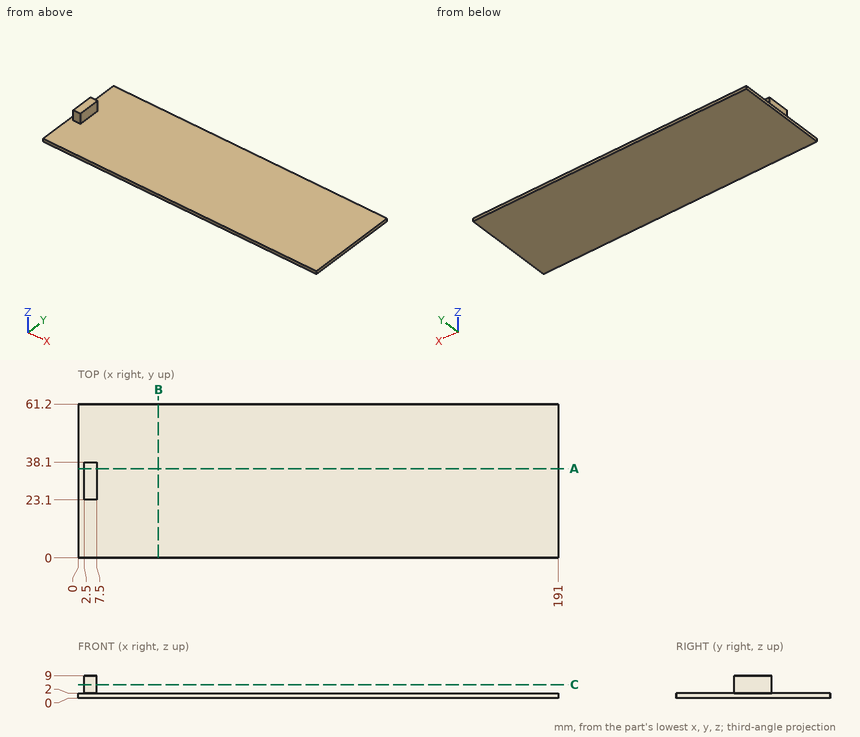
Check sheet for the drawn part. Datum: minimum x, y, z corner. Units: mm. Give positions to 0.01 mm unless a question says otherwise; leave off trailing zeros. Order: outer loops, then holes, each group sorted by start corner. A loop starts at its lowest first (then second) coordinate and runs counter-clockwise, first axis right, second up.
1. Sectioned sample at A-A (y = 35.5). Record the boundary of the cut face in (x, z).
Completed:
outline: (0, 0) - (191, 0) - (191, 2) - (7.5, 2) - (7.5, 9) - (2.5, 9) - (2.5, 2) - (0, 2) - close
2. Sectioned sample at B-B (x = 32). Record the boundary of the cut face in (y, z), then the cut area to 3 significant figures.
Completed:
outline: (0, 0) - (61.2, 0) - (61.2, 2) - (0, 2) - close
area: 122 mm2
3. Depth check by flat-ended pin: pin 1 (3 mm diameter, centred on x = 165, y = 39.5, fed in from -Z); pin 2 (2 mm diameter, centred on y = 28, z = 6.5, fed in from -X); pin 3 (2 mm diameter, centred on y = 34, z = 6, fed in from +X). Enter the tip coordinate at first touch or a pass-through.
Completed:
pin 1: stops at z = 0
pin 2: stops at x = 2.5
pin 3: stops at x = 7.5
4. Sectioned sample at C-C (z = 5.5). Record the boundary of the cut face in (x, y).
Completed:
outline: (2.5, 23.1) - (7.5, 23.1) - (7.5, 38.1) - (2.5, 38.1) - close
5. Scan lines: line 1 (X direction, y = 25, z = 3.5); line 2 (Z direction, x = 39.5, y = 43.5). Record each from-to range of solid material in increasing order.
Completed:
line 1: x = 2.5 to 7.5
line 2: z = 0 to 2
